from build123d import *

# Parameters (mm, degrees)
BOSS_EXTRUDE1_DEPTH      = 5
BOSS_EXTRUDE1_DEPTH_BACK = 5
SKETCH1_R                = 1.5
CUT_EXTRUDE1_DEPTH       = 5
SKETCH4_W                = 9.454278837
SKETCH4_H                = 9.25
CUT_EXTRUDE2_DEPTH       = 5


with BuildPart() as part:
    # Sketch1 → Boss-Extrude1 (new, two sides: drawn at the far end of the back side and taken through both)
    with BuildSketch(Plane(origin=(0, 0, 0), x_dir=(1, 0, 0), z_dir=(0, 1, 0)).offset(-BOSS_EXTRUDE1_DEPTH_BACK)):
        with BuildLine():
            Line((0, 22.5), (0, 36))
            Line((0, 36), (-36, 36))
            Line((-36, 36), (-36, -36))
            Line((-36, -36), (0, -36))
            Line((0, -36), (0, -22.5))
            ThreePointArc((0, -22.5), (-22.5, 0), (0, 22.5))
        make_face()
        with Locations(Location((-24.748737342, -24.748737342, 0), (0, 0, 270))):
            Circle(SKETCH1_R, mode=Mode.SUBTRACT)
        with Locations(Location((-24.748737342, 24.748737342, 0), (0, 0, 270))):
            Circle(SKETCH1_R, mode=Mode.SUBTRACT)
    extrude(amount=BOSS_EXTRUDE1_DEPTH + BOSS_EXTRUDE1_DEPTH_BACK)

    # Sketch2 → Cut-Extrude1 (cut)
    with BuildSketch(Plane(origin=(0, 5, 0), x_dir=(1, 0, 0), z_dir=(0, 1, 0))):
        Polygon((-23.161024101, 27.498737342), (-26.336450582, 27.498737342), (-27.924163822, 24.748737342), (-26.336450582, 21.998737342), (-23.161024101, 21.998737342), (-21.573310861, 24.748737342), align=None)
    cut_extrude1 = extrude(amount=-CUT_EXTRUDE1_DEPTH, mode=Mode.SUBTRACT)

    # Mirror1: Cut-Extrude1 across plane
    add(cut_extrude1.mirror(Plane.XY), mode=Mode.SUBTRACT)

    # Sketch4 → Cut-Extrude2 (cut)
    with BuildSketch(Plane.XZ.offset(5)):
        with Locations((-4.727139419, -29.25)):
            Rectangle(SKETCH4_W, SKETCH4_H)
    cut_extrude2 = extrude(amount=-CUT_EXTRUDE2_DEPTH, mode=Mode.SUBTRACT)

    # Mirror3: Cut-Extrude2 across plane
    add(cut_extrude2.mirror(Plane.XY), mode=Mode.SUBTRACT)


solid = part.part
Could you check a few things on this model? Use its own coordinates, in mm. A direction names the side the tool comes from. Coordinates: 2 decimals unless noted, no trailing zeros. Loops run counter-clockwise (first coordinate to the right, second up) from the corner with the lowest first, then second, coordinate; pieces in that order, holes last. Notation, with made-up numbers: (53.25, 56.25) -> (110.25, 56.25) arc R8 ccw to (110.25, 60.25) -> close; hole circle Ø9 at (10.5, 35). An arc over 180 degrees is marked (long way). Answer in a Markdown table with one row per item.
(1) Thinking about a two-plate mould opening in Z: for faces 1 (the face through (-23, 0, -25)), 2 (the face through (0, 2, -29)), 3 (the face through (-18, 0, -36)), which applies, released by +Z, released by -Z, zero draft, split by the parting line, or undercut?
Results found:
| item | result |
|---|---|
| face 1 | undercut |
| face 2 | zero draft |
| face 3 | released by -Z |
(2) If I drill on probe 1 along Z at (x, y) = (-9, -0.25) (3 decimals); probe 2 along Z at (x, y) = (-4, -3) (3 decimals); probe 3 along Y at (x, z) = (-5, -33), over which ranges is the centre line in solid material (lowest first)?
Results found:
| item | result |
|---|---|
| probe 1 | z = -36 to -33.875, -24.625 to -20.622, 20.622 to 24.625, 33.875 to 36 |
| probe 2 | z = -36 to -33.875, -24.625 to -22.142, 22.142 to 24.625, 33.875 to 36 |
| probe 3 | y = 0 to 5 |
(3) For faces 4 (the face through (-22.38, 2.54, 23.35)), 5 (the face through (-24.68, -2.54, 23.25)), 6 (the face through (-5, -3, 33.875)), which set-ups out of +Z, -Z, +X, -X, +Y, -Y let a thin tool reach every point of the face, with its end or its side?
Results found:
| item | result |
|---|---|
| face 4 | +Y |
| face 5 | +Y, -Y |
| face 6 | +X, -Y |
(4) Will these pins go through, and if not, where does the flat tip stop? pin 1 Ø8 at (x, z) = (-16.5, 5.5) entering from +Y; pin 2 Ø1.5 at (y, z) = (1.5, 13) entering from +X; pin 3 Ø4 at (x, z) = (-24.75, -24.75) entering from +Y; pin 4 Ø3 at (x, z) = (-4.5, -29.5) entering from -Y.
Results found:
| item | result |
|---|---|
| pin 1 | passes through |
| pin 2 | stops at x = -17.81 |
| pin 3 | stops at y = 0 |
| pin 4 | stops at y = 0 |
(5) Imagine slicing it at D-D (x = -11.5). List the corners of the cut face in (y, z) for me, plus the area to 3 significant figures.
Results found:
| item | result |
|---|---|
| outline | (-5, -36) -> (5, -36) -> (5, -19.34) -> (-5, -19.34) -> close; (-5, 19.34) -> (5, 19.34) -> (5, 36) -> (-5, 36) -> close |
| area | 333 mm^2 |
(6) Imagine slicing it at A-A (x = -25.5). List the corners of the cut face in (y, z) for me, plus the area to 3 significant figures.
Results found:
| item | result |
|---|---|
| outline | (-5, -36) -> (5, -36) -> (5, -27.5) -> (0, -27.5) -> (0, -26.05) -> (-5, -26.05) -> close; (-5, -23.45) -> (0, -23.45) -> (0, -22) -> (5, -22) -> (5, 22) -> (0, 22) -> (0, 23.45) -> (-5, 23.45) -> close; (-5, 26.05) -> (0, 26.05) -> (0, 27.5) -> (5, 27.5) -> (5, 36) -> (-5, 36) -> close |
| area | 639 mm^2 |
(7) Imagine slicing it at C-C (z = -32). List the corners of the cut face in (x, y) for me, plus the area to 3 significant figures.
Results found:
| item | result |
|---|---|
| outline | (-36, -5) -> (-9.45, -5) -> (-9.45, 0) -> (0, 0) -> (0, 5) -> (-36, 5) -> close |
| area | 313 mm^2 |
(8) Imagine slicing it at B-B (x = -6). List the corners of the cut face in (y, z) for me (3 decimals).
Results found:
| item | result |
|---|---|
| outline | (-5, -36) -> (5, -36) -> (5, -21.685) -> (-5, -21.685) -> (-5, -24.625) -> (0, -24.625) -> (0, -33.875) -> (-5, -33.875) -> close; (-5, 21.685) -> (5, 21.685) -> (5, 36) -> (-5, 36) -> (-5, 33.875) -> (0, 33.875) -> (0, 24.625) -> (-5, 24.625) -> close |
